Source: CAD feature listing. Evaluate the final solid. Frame: model axes, mm. Face numbers are marked on the shaded views. A direction names the side the tool comes from. Round coordinates to 2 decimals unless told otherwise and drop trailing zeros. Loops run counter-clockwise (first coordinate to the right, second up) from the corner with the lowest first, then second, coordinate; pieces in that order, holes last. Notation, with made-up numbers: (4, 20.5) - (22, 20.5) arc R22 ccw to (22, 37.5) - close; hole circle Ø8 at (-13.75, 4). An arc over 180 degrees is marked (long way). Use CSV: the item, a comma, the result in double quotes. Start each with the question number.
from build123d import *

# Parameters (mm, degrees)
SKETCH1_W           = 7.9
SKETCH1_H           = 13
BOSS_EXTRUDE1_DEPTH = 9.4
SKETCH2_W           = 2
SKETCH2_H           = 1.1
BOSS_EXTRUDE2_DEPTH = 4.5
SKETCH3_R           = 3.175
BOSS_EXTRUDE3_DEPTH = 8.9


with BuildPart() as part:
    # Sketch1 → Boss-Extrude1 (new body)
    with BuildSketch(Plane(origin=(0, 0, 0), x_dir=(1, 0, 0), z_dir=(0, 1, 0))):
        Rectangle(SKETCH1_W, SKETCH1_H)
    extrude(amount=-BOSS_EXTRUDE1_DEPTH)

    # Sketch2 → Boss-Extrude2 (add)
    with BuildSketch(Plane.XZ.offset(9.4)):
        with Locations((0, 4.7)):
            Rectangle(SKETCH2_W, SKETCH2_H)
        Rectangle(SKETCH2_W, SKETCH2_H)
    extrude(amount=BOSS_EXTRUDE2_DEPTH)

    # Sketch3 → Boss-Extrude3 (add)
    with BuildSketch(Plane(origin=(0, 0, 0), x_dir=(1, 0, 0), z_dir=(0, 1, 0))):
        with Locations(Location((0, 0, 0), (0, 0, 270))):
            Circle(SKETCH3_R)
    extrude(amount=BOSS_EXTRUDE3_DEPTH)

    # Sketch4 → Revolve1 (revolve)
    with BuildSketch(Plane(origin=(0, 0, 0), x_dir=(0, 0, -1), z_dir=(1, 0, 0)), mode=Mode.PRIVATE) as revolve1_sk:
        with BuildLine():
            Line((0, 8.9), (1.43399132, 8.9))
            Line((1.43399132, 8.9), (-0.960979548, 19.70301546))
            ThreePointArc((-0.960979548, 19.70301546), (-1.575574506, 20.580748024), (-2.630809417, 20.76681441))
            Line((-2.630809417, 20.76681441), (0, 8.9))
        make_face()
    revolve(revolve1_sk.sketch.rotate(Axis((0, 20.76681441, 2.630809417), (0, -0.9762960071199331, -0.21643961393810368)), 180), axis=Axis((0, 20.76681441, 2.630809417), (0, -0.9762960071199331, -0.21643961393810368)))


solid = part.part
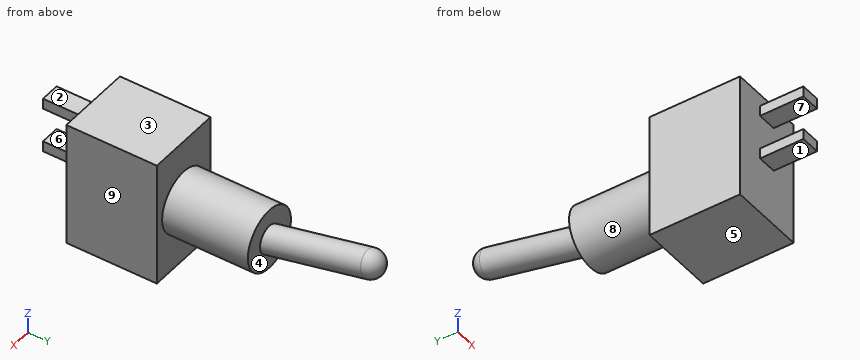
1. Contact query for flat-ended pins moving along their axis: P1, Ø1, axis at x = -0.5, y = -11, coming from the +Z side; P2, Ø3, axis at x = 1, y = 9, coming from the -Z side (3 decimals); P3, Ø0.6, axis at y = -11, z = 0, coming from the +X side. Output: stop coordinate, or through.
2. Section query D-D on x = 0. Return the cut outline in (y, z) (3 decimals).
3. Reachability of the marked faces 1, 2, 3, 4 and 5 from +Z, -Z, +X, -X, +Y, -Y: full face, straight path, thin tool, end or side. Return the list, or none.
4. Section query B-B on x = -2. Return the cut outline in (y, z).
5. Section query C-C on y = 7. Return the cut outline in (x, z) (3 decimals).
6. Mould query, pull axis Z, two halves, no side actions, for the marked faces 6, 7, 8 and 9. Classes: +Z half, -Z half, draft (parallel to the pull), parting line (faces both ways), or undercut.
7. Line query: line 1 along Y through (x, z) = (3, 2.25); line 2 along X through (y, z) = (16.5, 3); line 3 along Y through (x, z) = (2.25, -0.25). Output: solid intervals per line, ascending.
8. Section query A-A on z = 4.5. Return the cut outline in (x, y), and give its area (3 significant figures).
Values:
1,P1,"stops at z = 5.25"
1,P2,"stops at z = -3.175"
1,P3,"stops at x = 1"
2,outline,"(-13.9, -0.55) - (-9.4, -0.55) - (-9.4, -6.5) - (0, -6.5) - (0, -3.175) - (8.9, -3.175) - (8.9, -1.434) - (19.703, 0.961) arc R1.4 ccw to (19.097, 3.695) - (8.9, 1.434) - (8.9, 3.175) - (0, 3.175) - (0, 6.5) - (-9.4, 6.5) - (-9.4, 5.25) - (-13.9, 5.25) - (-13.9, 4.15) - (-9.4, 4.15) - (-9.4, 0.55) - (-13.9, 0.55) - close"
3,face 1,"-Z, +X, -X, -Y"
3,face 2,"+Z, +X, -X, -Y"
3,face 3,"+Z, +X, -X, +Y, -Y"
3,face 4,"none"
3,face 5,"-Z, +X, -X, +Y, -Y"
4,outline,"(-9.4, -6.5) - (0, -6.5) - (0, -2.47) - (8.9, -2.47) - (8.9, 2.47) - (0, 2.47) - (0, 6.5) - (-9.4, 6.5) - close"
5,outline,"circle Ø6.35 at (0, 0)"
6,face 6,"undercut"
6,face 7,"undercut"
6,face 8,"parting line"
6,face 9,"draft"
7,line 1,"y = -9.4 to 0"
7,line 2,"x = -0.56 to 0.56"
7,line 3,"y = -9.4 to 8.9"
8,outline,"(-3.95, -9.4) - (-1, -9.4) - (-1, -13.9) - (1, -13.9) - (1, -9.4) - (3.95, -9.4) - (3.95, 0) - (-3.95, 0) - close"
8,area,"83.3 mm^2"
